Here's how the part is built. I have some questions about the finished solid (model axes, mm). Face numbers are marked on the shaded views. A direction names the side the tool comes from. Round coordinates to 2 decimals unless told otherwise and drop trailing zeros. Use a Markdown table: item, result.
from build123d import *

# Parameters (mm, degrees)
F0_W     = 76.2
F0_H     = 50.8
F1_DEPTH = 3.175
F2_R     = 1.6558767695
F2_R_2   = 2.6518381977
F2_R_3   = 3.3103533059
F2_R_4   = 2.921000123
F2_R_5   = 1.5450229593
F2_R_6   = 1.9050003029
F2_R_7   = 2.2895237278
F2_R_8   = 2.9892250919
F2_R_9   = 2.9320238784
F3_DEPTH = 0.635
F5_DEPTH = 50.8


# Not quite as in the source:
# - a feature names something its author has since deleted; it is built from what else it names


with BuildPart() as f1:
    # F0 (on Front) → F1 (new body)
    with BuildSketch(Plane.XZ):
        with Locations((38.1, 25.4)):
            Rectangle(F0_W, F0_H)
    extrude(amount=F1_DEPTH)

    # F2 (on face) → F3 (cut)
    with BuildSketch(Plane.XZ.offset(3.175)):
        Polygon((48.691868487, 42.4682941364), (40.1828733117, 45.1352943044), (34.9758711487, 42.4682941364), (31.1658705429, 43.4842941893), (22.9070743114, 39.2204960176), (18.8385191247, 32.9432937858), (18.8385191247, 29.7757912988), (15.8623714775, 32.9432937858), (15.8623714775, 28.1172938255), (17.5768719597, 22.418530716), (23.9268724651, 14.5282934961), (20.4978712678, 14.5282934961), (27.3558708683, 10.0832957385), (30.27687006, 11.35329563), (37.1348724544, 10.0832957385), (43.2308704436, 12.7502943931), (43.2308704436, 8.1782940386), (45.7990180271, 10.59129495), (51.9938726753, 15.2902941761), (51.9938726753, 17.8302939592), (53.930624873, 20.4972944764), (53.930624873, 23.545293471), (55.0292181151, 22.418530716), (56.1848726899, 23.545293471), (58.6613714775, 21.005293688), (56.9468696446, 32.435293643), (55.1688742668, 35.356293766), (53.7718717784, 35.356293766), (51.9938726753, 36.8802941946), (45.7990180271, 40.1225700636), (45.3898717493, 41.4522940835), align=None)
        with Locations((27.9908708141, 16.1792937277)):
            Circle(F2_R, mode=Mode.SUBTRACT)
        with Locations((33.1978739083, 14.7822949646)):
            Circle(F2_R_2, mode=Mode.SUBTRACT)
        with Locations((22.1488724307, 25.3232944367)):
            Circle(F2_R_3, mode=Mode.SUBTRACT)
        with BuildLine():
            Line((29.4827647798, 21.2285935147), (28.6258707598, 26.5932943282))
            Line((28.6258707598, 26.5932943282), (30.4038726569, 24.1802934168))
            Line((30.4038726569, 24.1802934168), (31.6916008863, 24.6882943394))
            Line((31.6916008863, 24.6882943394), (32.4751487195, 22.7020840415))
            Line((32.4751487195, 22.7020840415), (34.7450423849, 23.8972995039))
            Line((34.7450423849, 23.8972995039), (33.3584630646, 26.5306218754))
            ThreePointArc((33.3584630646, 26.5306218754), (30.6271191315, 28.6945286164), (31.9278740168, 31.9272935001))
            ThreePointArc((31.9278740168, 31.9272935001), (32.188274126, 29.3087235679), (34.5948708088, 28.2442945597))
            Line((34.5948708088, 28.2442945597), (35.9297474949, 26.173913466))
            Line((35.9297474949, 26.173913466), (38.8855502865, 29.0062933771))
            ThreePointArc((38.8855502865, 29.0062933771), (41.5322516722, 29.6478879221), (43.484871912, 31.5462940914))
            ThreePointArc((43.484871912, 31.5462940914), (42.2018854798, 26.3705417725), (36.9460296513, 25.4702941614))
            Line((36.9460296513, 25.4702941614), (35.9297474949, 23.8972995039))
            Line((35.9297474949, 23.8972995039), (37.4565196476, 22.7832946537))
            Line((37.4565196476, 22.7832946537), (38.571963384, 23.8972995039))
            Line((38.571963384, 23.8972995039), (41.2807169848, 22.2783325716))
            Line((41.2807169848, 22.2783325716), (44.2106343052, 23.8972995039))
            Line((44.2106343052, 23.8972995039), (41.5642807871, 19.4857340033))
            Line((41.5642807871, 19.4857340033), (38.6588719517, 21.2285935147))
            Line((38.6588719517, 21.2285935147), (36.9460296513, 18.3732244384))
            Line((36.9460296513, 18.3732244384), (34.3611069299, 21.2285935147))
            Line((34.3611069299, 21.2285935147), (33.1806698754, 19.4857340033))
            Line((33.1806698754, 19.4857340033), (30.9118700058, 22.7832946537))
            Line((30.9118700058, 22.7832946537), (29.4827647798, 21.2285935147))
        make_face(mode=Mode.SUBTRACT)
        with Locations((46.1518705666, 17.1952940134)):
            Circle(F2_R_4, mode=Mode.SUBTRACT)
        with Locations((50.8508716554, 24.1802934168)):
            Circle(F2_R_5, mode=Mode.SUBTRACT)
        with Locations((22.9108707823, 31.0382939485)):
            Circle(F2_R_6, mode=Mode.SUBTRACT)
        with Locations((29.3878714398, 38.277293889)):
            Circle(F2_R_7, mode=Mode.SUBTRACT)
        with Locations((51.1048731238, 29.1332941113)):
            Circle(F2_R_8, mode=Mode.SUBTRACT)
        with Locations((39.4208707691, 38.658294229)):
            Circle(F2_R_9, mode=Mode.SUBTRACT)
    extrude(amount=-F3_DEPTH, mode=Mode.SUBTRACT)

    # F4 (on Top) → F5 (join)
    with BuildSketch(Plane.XY):
        with BuildLine():
            ThreePointArc((30.0156539358, 0), (38.1572704301, 8.1416164943), (46.2988869244, 0))
            Line((46.2988869244, 0), (48.7363704301, 0))
            ThreePointArc((48.7363704301, 0), (38.1572704301, 10.5791), (27.5781704301, 0))
            Line((27.5781704301, 0), (30.0156539358, 0))
        make_face()
    extrude(amount=F5_DEPTH)


solid = f1.part
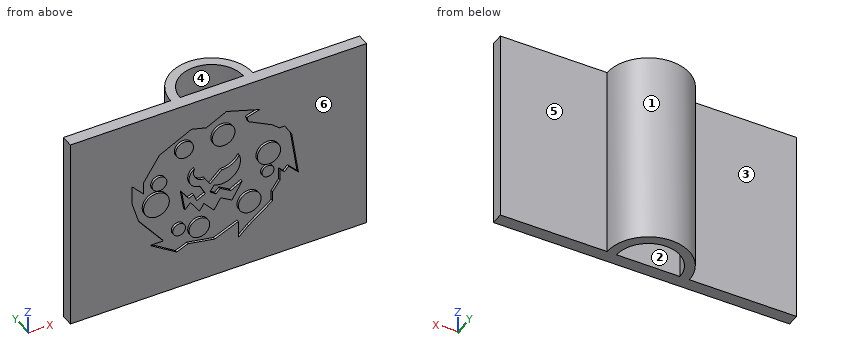
1. For pin 1 Ø4 at (y, z) = (4, 44.5) entering from -X; pin 2 Ø22 at (x, z) = (60.5, 27) entering from +Y; pin 3 Ø8 at (x, z) = (39, 27) entering from +Y; pin 4 Ø22 at (x, z) = (20.5, 19) entering from +Y, each with a flat end and sliding along its axis, tell me the tip position at first contact or that it passes through.
Answer sheet:
| item | result |
|---|---|
| pin 1 | x = 27.77 |
| pin 2 | y = 0 |
| pin 3 | y = 10.58 |
| pin 4 | y = 8.22 |
2. Which directions (+Z, -Z, +X, -X, +Y, -Y) give clear straight access to the entire face, cutting with the end or side of a thin tool? Please do the marked faces 4, 5 and 6.
Answer sheet:
| item | result |
|---|---|
| face 4 | +Z, -Z |
| face 5 | +Z, -Z, +X, +Y |
| face 6 | +Z, -Z, +X, -X, -Y |
3. We'd pull the mould along X, two halves only. Please class the marked faces 1, 2 and 3: +X half, -X half, draft (parallel to the pull), parting line (faces both ways), or undercut.
Answer sheet:
| item | result |
|---|---|
| face 1 | parting line |
| face 2 | undercut |
| face 3 | draft |
4. I need wall thicknesses on probe 1 along Y at (x, z) = (22, 21); probe 2 along Y at (x, z) = (63, 22.5) (3 decimals); probe 3 along X at (y, z) = (3, 33). Which ranges of each line are inside material? Lowest first, please. Write a range as from..to.
Answer sheet:
| item | result |
|---|---|
| probe 1 | -2.54..0 |
| probe 2 | -3.175..0 |
| probe 3 | 28.01..30.59, 45.73..48.3 |
